Autodesk Inventor part; units mm, degrees
ref_plane "YZ Plane" through (0, 0, 0) normal (1, 0, 0) x (0, 1, 0)
ref_plane "XZ Plane" through (0, 0, 0) normal (0, 1, 0) x (-1, 0, 0)
ref_plane "XY Plane" through (0, 0, 0) normal (0, 0, 1) x (1, 0, 0)
ref_plane "Work Plane1" through (0, 0, 0) normal (0, 0, 1) x (1, 0, 0)
sketch "Sketch1" plane through (0, 0, 0) normal (0, 0, 1) x (1, 0, 0)
  line L0 (-40, 0) -> (-40, 6)
  line L1 (-40, 6) -> (-34, 6)
  line L2 (0, 6) -> (-34, 6)
  line L3 (0, 6) -> (30, 6)
  line L4 (60, 6) -> (30, 6)
  line L5 (60, 6) -> (90, 6)
  line L6 (120, 6) -> (90, 6)
  line L7 (120, 6) -> (150, 6)
  line L8 (150, 6) -> (150, 0)
  line L9 (150, 0) -> (180, 0)
  line L10 (180, 0) -> (180, 6)
  line L11 (180, 6) -> (150, 6)
  line L12 (180, 6) -> (210, 6)
  line L13 (180, 0) -> (180, 6)
  line L14 (210, 0) -> (180, 0)
  line L15 (210, 0) -> (210, 6)
  line L16 (240, 0) -> (240, 6)
  line L17 (240, 6) -> (210, 6)
  line L18 (210, 6) -> (210, 0)
  line L19 (210, 0) -> (240, 0)
  line L20 (120, 6) -> (150, 6)
  line L21 (120, 0) -> (120, 6)
  line L22 (150, 0) -> (120, 0)
  line L23 (150, 0) -> (150, 6)
  line L24 (60, 6) -> (90, 6)
  line L25 (60, 0) -> (60, 6)
  line L26 (90, 0) -> (60, 0)
  line L27 (90, 0) -> (90, 6)
  line L28 (90, 6) -> (90, 0)
  line L29 (90, 0) -> (120, 0)
  line L30 (120, 0) -> (120, 6)
  line L31 (120, 6) -> (90, 6)
  line L32 (30, 6) -> (30, 0)
  line L33 (30, 0) -> (60, 0)
  line L34 (60, 0) -> (60, 6)
  line L35 (60, 6) -> (30, 6)
  line L36 (-34, 6) -> (-34, 0)
  line L37 (-34, 0) -> (0, 0)
  line L38 (0, 0) -> (0, 6)
  line L39 (0, 6) -> (-34, 6)
  line L40 (240, 0) -> (240, 6)
  line L41 (240, 6) -> (210, 6)
  line L42 (210, 6) -> (210, 0)
  line L43 (210, 0) -> (240, 0)
  line L44 (150, 6) -> (150, 0)
  line L45 (150, 0) -> (180, 0)
  line L46 (180, 0) -> (180, 6)
  line L47 (180, 6) -> (150, 6)
  line L48 (90, 6) -> (90, 0)
  line L49 (90, 0) -> (120, 0)
  line L50 (120, 0) -> (120, 6)
  line L51 (120, 6) -> (90, 6)
  line L52 (240, 6) -> (270, 6)
  line L53 (240, 0) -> (240, 6)
  line L54 (270, 0) -> (240, 0)
  line L55 (270, 0) -> (270, 6)
  line L56 (300, 0) -> (300, 6)
  line L57 (300, 6) -> (270, 6)
  line L58 (270, 6) -> (270, 0)
  line L59 (270, 0) -> (300, 0)
  line L60 (300, 6) -> (330, 6)
  line L61 (300, 0) -> (300, 6)
  line L62 (330, 0) -> (300, 0)
  line L63 (330, 0) -> (330, 6)
  line L64 (360, 0) -> (360, 6)
  line L65 (360, 6) -> (330, 6)
  line L66 (330, 6) -> (330, 0)
  line L67 (330, 0) -> (360, 0)
  line L68 (360, 6) -> (390, 6)
  line L69 (360, 0) -> (360, 6)
  line L70 (390, 0) -> (360, 0)
  line L71 (390, 0) -> (390, 6)
  line L72 (424, 0) -> (424, 6)
  line L73 (424, 6) -> (390, 6)
  line L74 (390, 6) -> (390, 0)
  line L75 (390, 0) -> (424, 0)
  line L76 (424, 6) -> (430, 6)
  line L77 (424, 0) -> (424, 6)
  line L78 (430, 0) -> (424, 0)
  line L79 (430, 6) -> (430, 0)
  line L80 (-40, 6) -> (-40, 21)
  line L81 (-40, 21) -> (430, 21)
  line L82 (430, 21) -> (430, 6)
  line L83 (0, 6) -> (30, 6)
  line L84 (0, 0) -> (0, 6)
  line L85 (30, 0) -> (0, 0)
  line L86 (30, 0) -> (30, 6)
  line L87 (-40, 6) -> (-34, 6)
  line L88 (-40, 0) -> (-40, 6)
  line L89 (-34, 0) -> (-40, 0)
  line L90 (-34, 0) -> (-34, 6)
  line L91 (-34, 6) -> (-34, 21)
  line L92 (424, 6) -> (424, 21)
  dimension "d0" = 15
extrude "Plate1" add sketch "Sketch1" along normal blind 6 contours L91 L81 L92 L73 L68 L65 L60 L57 L52 L17 L12 L11 L7 L6 L5 L4 L3 L2 | L38 L3 L32 L85 | L25 L5 L27 L26 | L71 L70 L64 L68 | L21 L7 L8 L22 | L63 L62 L56 L60 | L10 L12 L15 L14 | L55 L54 L16 L52
sketch "Sketch2" plane through (0, 0, 6) normal (0, 0, 1) x (1, 0, 0)
  line L0 (71.2707, 6) -> (65.2707, 6)
  line L1 (83.7293, 6) -> (77.7293, 6)
  line L2 (-34, 6) -> (-34, 21)
  line L3 (0, 6) -> (-34, 6)
  line L4 (0, 0) -> (0, 6)
  line L5 (30, 0) -> (0, 0)
  line L6 (30, 6) -> (30, 0)
  line L7 (60, 6) -> (30, 6)
  line L8 (60, 0) -> (60, 6)
  line L9 (90, 0) -> (60, 0)
  line L10 (90, 6) -> (90, 0)
  line L11 (120, 6) -> (90, 6)
  line L12 (120, 0) -> (120, 6)
  line L13 (150, 0) -> (120, 0)
  line L14 (150, 6) -> (150, 0)
  line L15 (180, 6) -> (150, 6)
  line L16 (180, 0) -> (180, 6)
  line L17 (210, 0) -> (180, 0)
  line L18 (210, 6) -> (210, 0)
  line L19 (240, 6) -> (210, 6)
  line L20 (240, 0) -> (240, 6)
  line L21 (270, 0) -> (240, 0)
  line L22 (270, 6) -> (270, 0)
  line L23 (300, 6) -> (270, 6)
  line L24 (300, 0) -> (300, 6)
  line L25 (330, 0) -> (300, 0)
  line L26 (330, 6) -> (330, 0)
  line L27 (360, 6) -> (330, 6)
  line L28 (360, 0) -> (360, 6)
  line L29 (390, 0) -> (360, 0)
  line L30 (390, 6) -> (390, 0)
  line L31 (424, 6) -> (390, 6)
  line L32 (424, 21) -> (424, 6)
  line L33 (-34, 21) -> (424, 21)
  line L34 (77.6, 6) -> (71.4, 6)
  line L35 (71.4, 6) -> (71.4, 12.2)
  line L36 (71.4, 12.2) -> (77.6, 12.2)
  line L37 (77.6, 12.2) -> (77.6, 6)
  line L38 (71.2707, 6) -> (77.7293, 6) construction
  point P0 (0, 0)
  point P1 (74.5, 6)
  point P2 (74.5, 6)
  dimension "d2" = 6.2
  dimension "d3" = 6.2
extrude "Cut1" cut sketch "Sketch2" against normal blind 6 contours L34 L35 L36 L37
equation "\"d3\" = d2"
equation "\"d4\" = Thickness"
equation "\"d1\" = Thickness"
equation "\"BendRadius\" = Thickness"
equation "\"BendReliefWidth\" = Thickness"
equation "\"BendReliefDepth\" = 0.5 * Thickness"
equation "\"CornerReliefSize\" = 4 * Thickness"
equation "\"MinimumRemnant\" = 2 * Thickness"
equation "\"TransitionRadius\" = BendRadius"
equation "\"JacobiRadiusSize\" = BendRadius"
equation "\"GapSize\" = Thickness"
properties part number "voorzijde onderkant elektrobox v2" material "Wood (Birch)"
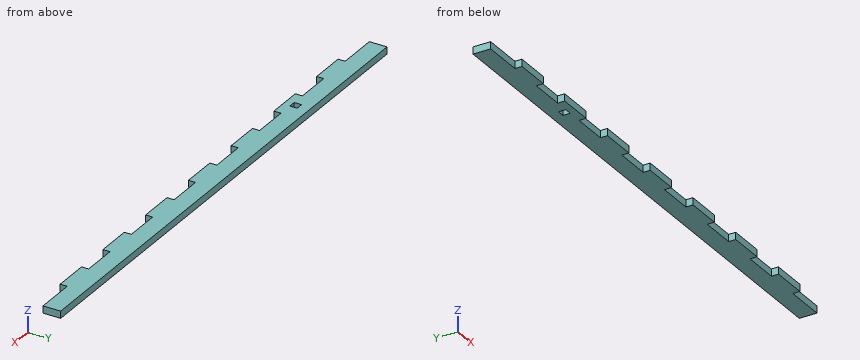
The listing builds one solid part. Answer for the finished solid, in the listing's coordinates (mm). Give positions to 0.01 mm unless a question says otherwise; leave off trailing zeros. Write each loop counter-clockwise with the first axis right and the second up, starting at its lowest first coordinate (ties: lowest second). Pieces come first, ordered by that corner, then holes.
1) Find the intervals of material crossed by L1, parallel to X at y = 11, z = 5.2; L2, parallel to Y at x = 75, z = 1.5; L3, parallel to Y at x = 165, z = 5.6, in increasing order.
2) Given P1, Ø1.8, axis at y = 2, z = 2.5, coming from the -X side; P2, Ø1.8, axis at y = 2.5, z = 4.5, coming from the +X side; P3, Ø3, axis at x = 401, z = 2, coming from the -Y side, each flat-ended and moving along its own axis, determine where each tip first touches the part or whether it passes through.
3) Section A-A (x = 219) is taken. Write down the section's boundary in (y, z).
Response:
1. L1: x = -34 to 71.4, 77.6 to 424
1. L2: y = 0 to 6, 12.2 to 21
1. L3: y = 6 to 21
2. P1: stops at x = 0
2. P2: stops at x = 390
2. P3: stops at y = 6
3. outline: (6, 0) - (21, 0) - (21, 6) - (6, 6) - close
